The model under review builds one solid part; all positions refer to its coordinate system, in mm. Face numbers are marked on the shaded views. A direction names the side the tool comes from. Coordinates: 2 decimals unless noted, no trailing zeros. Write each loop counter-clockwise with the first axis right and the second up, starting at its lowest first coordinate (ties: lowest second). Pieces come first, ordered by that corner, then holes. Notation, with made-up numbers: (56.25, 84) - (75.25, 84) arc R27 ccw to (75.25, 119) - close; hole circle Ø3 at (-24, 0.25). An arc over 180 degrees is marked (long way). Return JSON: item names as keys, results as strings. Group by question number.
(1) We need section C-C on z = 4.75. State the section outline as (x, y) points, then the cut area to 3 significant figures.
(2) We need section B-B on y = 27. State the section outline as (x, z) points.
(3) To check wall thickness, follow L1, parallel to X at y = 24.5, z = 18.75; L2, parallel to Y at x = -24, z = 10.5; L3, parallel to X at y = -28, z = 20.25. State the ranges of each line that lie inside material, in increasing order. Write a range as from..to.
(4) Draft analysis for pull direction X (two halves, no side actions). For the marked faces 1, 2 and 3, state which applies: released by +X, released by -X, zero draft, split by the parting line, or undercut.
(5) Tool access review of the marked faces 4, 5 and 6: name each direction out of +Z, -Z, +X, -X, +Y, -Y from which nothing blocks a thin tool from reaching the whole face with its end or side.
(6) We need section A-A on x = 27. State the section outline as (y, z) points.
(7) For pin 1 Ø4 at (x, z) = (-21, 15.5) entering from -Y; pin 2 Ø13 at (y, z) = (-53.5, 13.5) entering from -X, all flat-tipped, find the tip position at first contact; note any pin that passes through.
```python
from build123d import *

# Parameters (mm, degrees)
F0_R     = 15
F0_R_2   = 5
F0_R_3   = 25
F1_DEPTH = 25


with BuildPart() as f1:
    # F0 (on Top) → F1 (new body)
    with BuildSketch(Plane.XY):
        with BuildLine():
            Line((-29.817205, 54.56318), (-53.817205, 42.56318))
            Line((-53.817205, 42.56318), (-53.817205, -45.43682))
            Line((-53.817205, -45.43682), (-13.817205, -45.43682))
            Line((-13.817205, -45.43682), (-13.817205, -61.901286))
            Line((-13.817205, -61.901286), (-10.281671, -65.43682))
            Line((-10.281671, -65.43682), (102.647265, -65.43682))
            Line((102.647265, -65.43682), (106.182795, -61.90129))
            Line((106.182795, -61.90129), (106.182795, -45.43682))
            Line((106.182795, -45.43682), (146.182795, -45.43682))
            Line((146.182795, -45.43682), (146.182795, 29.56318))
            ThreePointArc((146.182795, 29.56318), (138.860464, 47.240849), (121.182795, 54.56318))
            Line((121.182795, 54.56318), (41.182795, 54.56318))
            Line((41.182795, 54.56318), (-29.817205, 54.56318))
        make_face()
        with Locations((-23.817205, -15.43682)):
            Circle(F0_R, mode=Mode.SUBTRACT)
        with Locations((126.182795, -30.43682)):
            Circle(F0_R_2, mode=Mode.SUBTRACT)
        with Locations((41.182795, 24.56318)):
            Circle(F0_R_3, mode=Mode.SUBTRACT)
    extrude(amount=F1_DEPTH)


solid = f1.part
```
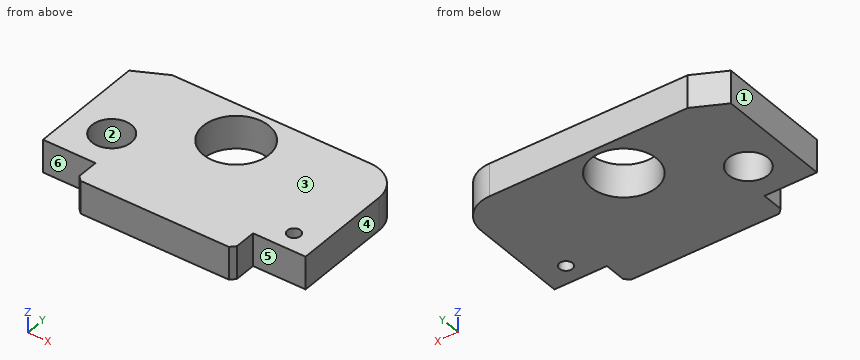
Ans:
{
 "1": {"outline": "(-53.82, -45.44) - (-13.82, -45.44) - (-13.82, -61.9) - (-10.28, -65.44) - (102.65, -65.44) - (106.18, -61.9) - (106.18, -45.44) - (146.18, -45.44) - (146.18, 29.56) arc R25 ccw to (121.18, 54.56) - (-29.82, 54.56) - (-53.82, 42.56) - close; hole circle Ø30 at (-23.82, -15.44); hole circle Ø50 at (41.18, 24.56); hole circle Ø10 at (126.18, -30.44)", "area": "19,400 mm²"},
 "2": {"outline": "(-53.82, 0) - (16.3, 0) - (16.3, 25) - (-53.82, 25) - close; (66.06, 0) - (146.18, 0) - (146.18, 25) - (66.06, 25) - close"},
 "3": {"L1": "-53.82..16.18, 66.18..146.18", "L2": "-45.44..-30.44, -0.44..54.56", "L3": "-53.82..-32.01, -15.62..121.82, 130.55..146.18"},
 "4": {"face 1": "released by -X", "face 2": "undercut", "face 3": "zero draft"},
 "5": {"face 4": "+Z, -Z, +X, +Y, -Y", "face 5": "+Z, -Z, +X, -Y", "face 6": "+Z, -Z, -X, -Y"},
 "6": {"outline": "(-65.44, 0) - (3.98, 0) - (3.98, 25) - (-65.44, 25) - close; (45.15, 0) - (54.56, 0) - (54.56, 25) - (45.15, 25) - close"},
 "7": {"pin 1": "y = -45.44", "pin 2": "x = -13.82"}
}
